Read the model definition and answer for the solid it produces. Units are mm, in the model's axes. A direction names the side the tool comes from. Give positions to 0.01 mm unless a question says otherwise; leave off trailing zeros. Order: outer loops, then holes, each group sorted by start corner. A loop starts at its lowest first (then second) coordinate and runs counter-clockwise, first axis right, second up. Notation, with made-up numbers: (61.25, 29.25) - (106.25, 29.25) arc R7 cw to (106.25, 35.25) - close; hole circle Ø7 at (30.25, 2). An arc over 180 degrees is marked (long way). Write each question's results on one line, items separated by ' | '.
from build123d import *

# Parameters (mm, degrees)
BOSS_EXTRUDE1_DEPTH     = 5
SKETCH2_R               = 15
BOSS_EXTRUDE2_DEPTH     = 2.5
SKETCH3_R               = 6
SKETCH3_W               = 4
SKETCH3_H               = 3.6
CUT_EXTRUDE1_DEPTH      = 6
CUT_EXTRUDE1_DEPTH_BACK = 3.5
FILLET2_R               = 0.25
FILLET1_R               = 1


with BuildPart() as part:
    # Sketch1 → Boss-Extrude1 (new body)
    with BuildSketch(Plane.XY):
        with BuildLine():
            ThreePointArc((11.187046571, 6.27376313), (9.091843201, 6.605610744), (9.423690814, 8.700814114))
            Line((9.423690814, 8.700814114), (19.307308392, 15.881682614))
            ThreePointArc((19.307308392, 15.881682614), (17.777891388, 17.576876224), (16.100198302, 19.125470312))
            ThreePointArc((16.100198302, 19.125470312), (5.786474508, 17.808937333), (-1.783664646, 24.936289628))
            ThreePointArc((-1.783664646, 24.936289628), (-4.051187632, 24.669573948), (-6.284921782, 24.197102268))
            Line((-6.284921782, 24.197102268), (-2.5097158, 12.578212966))
            ThreePointArc((-2.5097158, 12.578212966), (-3.472775082, 10.6881027), (-5.362885348, 11.651161982))
            Line((-5.362885348, 11.651161982), (-9.138091331, 23.270051285))
            ThreePointArc((-9.138091331, 23.270051285), (-11.222932105, 22.339332912), (-13.214168279, 21.22229386))
            ThreePointArc((-13.214168279, 21.22229386), (-15.149186938, 11.006528575), (-24.267003431, 6.009371387))
            ThreePointArc((-24.267003431, 6.009371387), (-24.714044883, 3.770409198), (-24.954959427, 1.5))
            Line((-24.954959427, 1.5), (-12.738136237, 1.5))
            ThreePointArc((-12.738136237, 1.5), (-11.238136237, 0), (-12.738136237, -1.5))
            Line((-12.738136237, -1.5), (-24.954959427, -1.5))
            ThreePointArc((-24.954959427, -1.5), (-24.714044883, -3.770409198), (-24.267003431, -6.009371387))
            ThreePointArc((-24.267003431, -6.009371387), (-15.149186938, -11.006528575), (-13.214168279, -21.22229386))
            ThreePointArc((-13.214168279, -21.22229386), (-11.222932105, -22.339332912), (-9.138091331, -23.270051285))
            Line((-9.138091331, -23.270051285), (-5.362885348, -11.651161982))
            ThreePointArc((-5.362885348, -11.651161982), (-3.472775082, -10.6881027), (-2.5097158, -12.578212966))
            Line((-2.5097158, -12.578212966), (-6.284921782, -24.197102268))
            ThreePointArc((-6.284921782, -24.197102268), (-4.051187632, -24.669573948), (-1.783664646, -24.936289628))
            ThreePointArc((-1.783664646, -24.936289628), (5.786474508, -17.808937333), (16.100198302, -19.125470312))
            ThreePointArc((16.100198302, -19.125470312), (17.777891388, -17.576876224), (19.307308392, -15.881682614))
            Line((19.307308392, -15.881682614), (9.423690814, -8.700814114))
            ThreePointArc((9.423690814, -8.700814114), (9.091843201, -6.605610744), (11.187046571, -6.27376313))
            Line((11.187046571, -6.27376313), (21.070664149, -13.454631631))
            ThreePointArc((21.070664149, -13.454631631), (22.210273232, -11.47622599), (23.164638055, -9.402103157))
            ThreePointArc((23.164638055, -9.402103157), (18.725424859, 0), (23.164638055, 9.402103157))
            ThreePointArc((23.164638055, 9.402103157), (22.210273232, 11.47622599), (21.070664149, 13.454631631))
            Line((21.070664149, 13.454631631), (11.187046571, 6.27376313))
        make_face()
    extrude(amount=BOSS_EXTRUDE1_DEPTH)

    # Sketch2 → Boss-Extrude2 (add)
    with BuildSketch(Plane.XY):
        Circle(SKETCH2_R)
    extrude(amount=-BOSS_EXTRUDE2_DEPTH)

    # Sketch3 → Cut-Extrude1 (cut, two sides)
    with BuildSketch(Plane.XY) as cut_extrude1_sk:
        Circle(SKETCH3_R)
        with Locations((0, 6)):
            Rectangle(SKETCH3_W, SKETCH3_H)
    extrude(amount=CUT_EXTRUDE1_DEPTH, mode=Mode.SUBTRACT)
    extrude(cut_extrude1_sk.sketch, amount=-CUT_EXTRUDE1_DEPTH_BACK, mode=Mode.SUBTRACT)

    # Fillet2
    fillet2_edges = [part.edges().sort_by_distance(p)[0] for p in [
        (-2, 7.8, 1.25),
        (2, 7.8, 1.25),
    ]]
    fillet(fillet2_edges, radius=FILLET2_R)

    # Fillet1
    fillet1_edges = [part.edges().sort_by_distance(p)[0] for p in [
        (-6.284921782, 24.197102268, 2.5),
        (-1.783664646, 24.936289628, 2.5),
        (16.100198302, 19.125470312, 2.5),
        (19.307308392, 15.881682614, 2.5),
        (21.070664149, 13.454631631, 2.5),
        (23.164638055, 9.402103157, 2.5),
        (23.164638055, -9.402103157, 2.5),
        (21.070664149, -13.454631631, 2.5),
        (19.307308392, -15.881682614, 2.5),
        (16.100198302, -19.125470312, 2.5),
        (-1.783664646, -24.936289628, 2.5),
        (-6.284921782, -24.197102268, 2.5),
        (-9.138091331, -23.270051285, 2.5),
        (-13.214168279, -21.22229386, 2.5),
        (-24.267003431, -6.009371387, 2.5),
        (-24.954959427, -1.5, 2.5),
        (-24.954959427, 1.5, 2.5),
        (-24.267003431, 6.009371387, 2.5),
        (-13.214168279, 21.22229386, 2.5),
        (-9.138091331, 23.270051285, 2.5),
    ]]
    fillet(fillet1_edges, radius=FILLET1_R)


solid = part.part
(1) Consider probe 1 along Y at (x, z) = (0, -0.25); probe 2 along X at (y, z) = (0, 1.5); probe 3 along X at (y, z) = (12, 4). Determine where each line is inside the solid, lowest interval first. Write a range as [from, to].
Conclusion:
probe 1: [-15, -6], [7.8, 15] | probe 2: [-11.24, -6], [6, 18.73] | probe 3: [-14.5, -5.48], [-2.44, 13.96], [19.07, 21.93]
(2) Each of these flat-tipped pins is pushed along its axis until it touches: pin 1 (7.5 mm diameter, centred on x = 3, y = 19.5, fed in from -Z); pin 2 (3 mm diameter, centred on x = -11.5, z = 3, fed in from +Y); pin 3 (3 mm diameter, centred on y = -5.5, z = 2, fed in from -X). Where does it stop, or does it pass through?
Conclusion:
pin 1: z = 0 | pin 2: y = 22.9 | pin 3: x = -24.68
(3) Section A-A (y = 0) is taken. Give the vertices of the cut face in (x, z), plus the area to 3 significant figures.
Conclusion:
outline: (-15, -2.5) - (-6, -2.5) - (-6, 5) - (-11.24, 5) - (-11.24, 0) - (-15, 0) - close; (6, -2.5) - (15, -2.5) - (15, 0) - (18.73, 0) - (18.73, 5) - (6, 5) - close | area: 135 mm^2
(4) The mould has two halves that part along Y. Classify faces 1 (the face through (17.634, -17.721, 2.465)), 2 (the face through (-15.233, -10.893, 2.465)), 3 (the face through (-13, 0, 0)), 4 (the face through (-0.2, -6.5, -2.5)): pulls with the +Y half, pulls with the -Y half, needs draft (parallel to the pull), parting line crosses it, or undercut.
Conclusion:
face 1: pulls with the -Y half | face 2: undercut | face 3: undercut | face 4: needs draft
(5) Section D-D (x = -9.5) is taken. Give the vertices of the cut face in (y, z), plus the area to 3 significant figures.
Conclusion:
outline: (-22.9, 0) - (-11.61, 0) - (-11.61, -2.5) - (11.61, -2.5) - (11.61, 0) - (22.9, 0) - (22.9, 5) - (-22.9, 5) - close | area: 287 mm^2
(6) Section B-B (x = 0) is taken. Give the vertices of the cut face in (y, z).
Conclusion:
outline: (-21.83, 0) - (-15, 0) - (-15, -2.5) - (-6, -2.5) - (-6, 5) - (-21.83, 5) - close; (7.8, -2.5) - (15, -2.5) - (15, 0) - (21.83, 0) - (21.83, 5) - (7.8, 5) - close
(7) Section C-C (x = -19) is taken. Give the vertices of the cut face in (y, z).
Conclusion:
outline: (-7.57, 0) - (-1.5, 0) - (-1.5, 5) - (-7.57, 5) - close; (1.5, 0) - (7.57, 0) - (7.57, 5) - (1.5, 5) - close
(8) For faces 5 (the face through (-14.985, 0.66, -1.232)), 6 (the face through (-14, 11, 0)), 7 (the face through (-5.86, -23.98, 2.54)), 8 (the face through (-18, 1.5, 2)), 9 (the face through (-4, -13, 0)), determine the directions among +Z, -Z, +X, -X, +Y, -Y from which every point of the face is accessible in a straight line to the end or side of a thin tool.
Conclusion:
face 5: -Z | face 6: -Z, -X, +Y | face 7: +Z, -Z, -X | face 8: +Z, -X | face 9: +Z
